The model under review builds one solid part; all positions refer to its coordinate system, in mm. A direction names the side the tool comes from. Round coordinates to 2 decimals unless told otherwise and drop trailing zeros. Order: outer loops, then holes, each group sorted by start corner. A loop starts at its lowest first (then second) coordinate and runs counter-clockwise, first axis right, second up. Notation, with made-up numbers: M 82,61 L 113,61 A21 ccw 113,87 Z; hole C -28.5,-17.5 d3. An arc over 180 degrees is marked long. Answer as a JSON object with one key per item and string values. Group by question number.
1. Add section C-C on y = 3. State the section outline as (x, z) points, and give its area (3 significant figures).
2. Machinability: for faces 1 (the face through (2.557, 2.192, -4.214)), 2 (the face through (1, 0, 1.5)), which of the approach directions +Z, -Z, +X, -X, +Y, -Y give a long, thin tool a straight path to every point of the face, cutting with its end or side? Answer none if there is none.
3. Add section B-B on z = 4. State the section outline as (x, y) points.
4. To check wall thickness, follow probe 1 along Y at (x, z) = (10.75, -1.75); probe 2 along X at (y, z) = (0.5, 3.75); probe 3 along Z at (x, y) = (8, 0). State the ranges of each line that lie inside material, in increasing order. Write a range as [from, to].
5. Clearance check with flat-ended pins moving along their axes: P1, Ø2, axis at x = 3.5, y = -3, coming from the -Z side; P2, Ø4, axis at x = 7.5, y = 0, coming from the +Z side; P3, Ø0.6, axis at y = -0.5, z = 1, coming from the -X side. State where each tip first meets the part, or that it passes through.
6. Add section A-A on x = 12.25. State the section outline as (y, z) points, and give its area (3 significant figures).
7. Mouldability with a two-part tool opening along Z and no side actions: class faces 3 (the face through (8.55, -0.54, -2.44)), 4 (the face through (2.75, -2.04, -2.04)), 5 (the face through (2.288, -0.19, -0.146)) as released by +Z, released by -Z, zero draft, split by the parting line, or undercut.
```python
from build123d import *

# Parameters (mm, degrees)
FILLET1_R   = 0.2
HEX_2_DEPTH = 1.56


with BuildPart() as part:
    # BodySke → BaseBody (revolve)
    with BuildSketch(Plane.XY):
        with BuildLine():
            Line((14.75, 0), (14.75, 2.055))
            Line((14.75, 2.055), (14.305, 2.5))
            Line((14.305, 2.5), (2.75, 2.5))
            Line((2.75, 2.5), (2.75, 4.75))
            Line((2.75, 4.75), (2.37, 4.75))
            ThreePointArc((2.37, 4.75), (0.992680215, 3.754414901), (0, 2.375))
            Line((0, 2.375), (0, 0))
            Line((0, 0), (14.75, 0))
        make_face()
    revolve(axis=Axis((0, 0, 0), (1, 0, 0)))

    # Fillet1
    fillet1_edges = [part.edges().sort_by_distance(p)[0] for p in [
        (2.75, -2.5, 0),
    ]]
    fillet(fillet1_edges, radius=FILLET1_R)

    # Sketch2 → PreBroach (revolve, cut)
    with BuildSketch(Plane.XY):
        Polygon((0, 1.5), (1.56, 1.5), (2.426025404, 0), (0, 0), align=None)
    revolve(axis=Axis((0, 0, 0), (1, 0, 0)), mode=Mode.SUBTRACT)

    # Sketch3 → Hex 2 (cut)
    with BuildSketch(Plane(origin=(0, 0, 0), x_dir=(0, 0, -1), z_dir=(1, 0, 0))):
        Polygon((-1.5, -0.866025404), (-1.5, 0.866025404), (0, 1.732050808), (1.5, 0.866025404), (1.5, -0.866025404), (0, -1.732050808), align=None)
    extrude(amount=HEX_2_DEPTH, mode=Mode.SUBTRACT)


solid = part.part
```
Recorded:
{
 "1": {"outline": "M 2.37,-3.68 L 2.75,-3.68 L 2.75,3.68 L 2.37,3.68 A4.39 ccw Z", "area": "13.2 mm²"},
 "2": {"face 1": "+X, -X", "face 2": "-X"},
 "3": {"outline": "M 2.37,-2.56 L 2.75,-2.56 L 2.75,2.56 L 2.37,2.56 A3.5 ccw Z"},
 "4": {"probe 1": "y = [-1.79, 1.79]", "probe 2": "x = [1.02, 2.75]", "probe 3": "z = [-2.5, 2.5]"},
 "5": {"P1": "stops at z = -4.13", "P2": "stops at z = 2.5", "P3": "stops at x = 1.61"},
 "6": {"outline": "C 0,0 d5", "area": "19.6 mm²"},
 "7": {"face 3": "split by the parting line", "face 4": "zero draft", "face 5": "undercut"}
}
